The listing builds one solid part. Answer for the finished solid, in the listing's coordinates (mm). Give positions to 0.01 mm unless a question says otherwise; leave off trailing zeros. Order: outer loops, then holes, each group sorted by start corner. A loop starts at its lowest first (then second) coordinate and runs counter-clockwise, first axis right, second up. Notation, with made-up numbers: (23.5, 51) - (70.5, 51) arc R34 cw to (70.5, 90) - close; hole circle Ø9 at (-30, 8.5). An arc over 180 degrees is marked (long way). Answer as a JSON object with one key per item and string values. Group by question number.
Q1. A cutting plane is placed at A-A, the plane y = 7.5. Give the vertices of the cut face in (x, z).
Q2. The mould has two halves that part along Y. Classify faces 1 (the face through (0.07, -14.14, 0.9)), 2 (the face through (0, 4, 5)), 3 (the face through (0, -10, 19)), 4 (the face through (0, 6, 3)): released by +Y, released by -Y, zero draft, split by the parting line, or undercut.
Q3. Consider line 1 (Y direction, x = 0, z = 3.95); line 2 (Z direction, x = 2.75, y = 5.75); line 3 (Y direction, x = 0, z = 1.9). Determine where each line is inside the solid, lowest interval first.
Q4. A cutting plane is placed at D-D, the plane x = -3. Give the vertices of the cut face in (y, z).
Q5. A cutting plane is placed at B-B, the plane x = 0. Give the vertices of the cut face in (y, z).
Q6. A cutting plane is placed at C-C, the plane z = 22.5. Give the vertices of the cut face in (x, y), and give its area (3 significant figures).
Q7. Given pin 1 (5 mm diameter, centred on x = -0.5, z = 21.5, fed in from +Y); pin 2 (5 mm diameter, centred on x = 0, y = 7.5, fed in from +Z), each flat-ended and moving along its own axis, determine where each tip first touches the part or whether it passes through.
from build123d import *

# Parameters (mm, degrees)
ESQUISSE1_W             = 10
ESQUISSE1_H             = 30
BOSS_EXTRU_1_DEPTH      = 5
ESQUISSE2_W             = 10
ESQUISSE2_H             = 5
BOSS_EXTRU_2_DEPTH      = 25
ESQUISSE3_R             = 1.5
ENL_V_MAT_EXTRU_1_DEPTH = 30
ESQUISSE4_R             = 1.5
ENL_V_MAT_EXTRU_2_DEPTH = 30
CONG_1_RADIUS           = 5
CONG_1_LENGTH           = 5
CONG_2_RADIUS           = 5
CONG_2_LENGTH           = 5
CONG_3_R                = 3
CONG_4_R                = 3


with BuildPart() as part:
    # Esquisse1 → Boss.-Extru.1 (new body)
    with BuildSketch(Plane.XY):
        Rectangle(ESQUISSE1_W, ESQUISSE1_H)
    extrude(amount=BOSS_EXTRU_1_DEPTH)

    # Esquisse2 → Boss.-Extru.2 (add)
    with BuildSketch(Plane.XY.offset(5)):
        with Locations((0, -12.5)):
            Rectangle(ESQUISSE2_W, ESQUISSE2_H)
    extrude(amount=BOSS_EXTRU_2_DEPTH)

    # Esquisse3 → Enlèv. mat.-Extru.1 (cut)
    with BuildSketch(Plane.XY.offset(5)):
        with Locations((0, 7.5)):
            Circle(ESQUISSE3_R)
    extrude(amount=-ENL_V_MAT_EXTRU_1_DEPTH, mode=Mode.SUBTRACT)

    # Esquisse4 → Enlèv. mat.-Extru.2 (cut)
    with BuildSketch(Plane(origin=(0, -10, 0), x_dir=(1, 0, 0), z_dir=(0, 1, 0))):
        with Locations(Location((0, -22.5, 0), (0, 0, 270))):
            Circle(ESQUISSE4_R)
    extrude(amount=-ENL_V_MAT_EXTRU_2_DEPTH, mode=Mode.SUBTRACT)

    # Congé1: full round fillet: the end face becomes a half cylinder, R = half its width
    cong_1_face = Plane((0, 15, 2.5), x_dir=(0, 0, 1), z_dir=(0, 1, 0))  # on the end face: x along it, z out of the body
    cong_1_slab = cong_1_face.offset(-CONG_1_RADIUS / 2) * Box(CONG_1_LENGTH, 2 * CONG_1_RADIUS, CONG_1_RADIUS, mode=Mode.PRIVATE)  # the body's end, R deep
    cong_1_round = Plane((0, 10, 2.5), x_dir=(0, 1, 0), z_dir=(0, 0, 1)) * Cylinder(CONG_1_RADIUS, CONG_1_LENGTH, mode=Mode.PRIVATE)  # its axis R under the face
    add(cong_1_slab - cong_1_round, mode=Mode.SUBTRACT)

    # Congé2: full round fillet: the end face becomes a half cylinder, R = half its width
    cong_2_face = Plane((0, -12.5, 30), x_dir=(0, 1, 0), z_dir=(0, 0, 1))  # on the end face: x along it, z out of the body
    cong_2_slab = cong_2_face.offset(-CONG_2_RADIUS / 2) * Box(CONG_2_LENGTH, 2 * CONG_2_RADIUS, CONG_2_RADIUS, mode=Mode.PRIVATE)  # the body's end, R deep
    cong_2_round = Plane((0, -12.5, 25), x_dir=(0, 0, 1), z_dir=(0, 1, 0)) * Cylinder(CONG_2_RADIUS, CONG_2_LENGTH, mode=Mode.PRIVATE)  # its axis R under the face
    add(cong_2_slab - cong_2_round, mode=Mode.SUBTRACT)

    # Congé3
    cong_3_edges = [part.edges().sort_by_distance(p)[0] for p in [
        (0, -15, 0),
    ]]
    fillet(cong_3_edges, radius=CONG_3_R)

    # Congé4
    cong_4_edges = [part.edges().sort_by_distance(p)[0] for p in [
        (0, -10, 5),
    ]]
    fillet(cong_4_edges, radius=CONG_4_R)


solid = part.part
Reply:
{
 "1": {"outline": "(-5, 0) - (-1.5, 0) - (-1.5, 5) - (-5, 5) - close; (1.5, 0) - (5, 0) - (5, 5) - (1.5, 5) - close"},
 "2": {"face 1": "released by -Y", "face 2": "zero draft", "face 3": "released by +Y", "face 4": "undercut"},
 "3": {"line 1": "y = -15 to 6, 9 to 15", "line 2": "z = 0 to 5", "line 3": "y = -14.79 to 6, 9 to 15"},
 "4": {"outline": "(-15, 3) arc R3 ccw to (-12, 0) - (14, 0) - (14, 5) - (-7, 5) arc R3 cw to (-10, 8) - (-10, 29) - (-15, 29) - close"},
 "5": {"outline": "(-15, 3) arc R3 ccw to (-12, 0) - (6, 0) - (6, 5) - (-7, 5) arc R3 cw to (-10, 8) - (-10, 21) - (-15, 21) - close; (-15, 24) - (-10, 24) - (-10, 30) - (-15, 30) - close; (9, 0) - (15, 0) - (15, 5) - (9, 5) - close"},
 "6": {"outline": "(-5, -15) - (-1.5, -15) - (-1.5, -10) - (-5, -10) - close; (1.5, -15) - (5, -15) - (5, -10) - (1.5, -10) - close", "area": "35.0 mm^2"},
 "7": {"pin 1": "stops at y = -10", "pin 2": "stops at z = 5"}
}
